from build123d import *

# Parameters (mm, degrees)
SKETCH1_R           = 3
SKETCH1_R_2         = 2.25
SKETCH1_W           = 9.525
SKETCH1_H           = 3.175
BOSS_EXTRUDE1_DEPTH = 3.175


with BuildPart() as part:
    # Sketch1 → Boss-Extrude1 (new body)
    with BuildSketch(Plane(origin=(0, 0, 0), x_dir=(1, 0, 0), z_dir=(0, 1, 0))):
        with BuildLine():
            Line((-12.7, -15.875), (101.8, -15.875))
            ThreePointArc((101.8, -15.875), (110.638834765, -12.213834765), (114.3, -3.375))
            Line((114.3, -3.375), (114.3, 3.375))
            ThreePointArc((114.3, 3.375), (110.638834765, 12.213834765), (101.8, 15.875))
            Line((101.8, 15.875), (-12.7, 15.875))
            Line((-12.7, 15.875), (-12.7, -15.875))
        make_face()
        Circle(SKETCH1_R, mode=Mode.SUBTRACT)
        with Locations((98.425, 0)):
            Circle(SKETCH1_R_2, mode=Mode.SUBTRACT)
        with Locations((50.8, 0)):
            Circle(SKETCH1_R, mode=Mode.SUBTRACT)
        with Locations((12.7, 0)):
            Rectangle(SKETCH1_W, SKETCH1_H, mode=Mode.SUBTRACT)
    extrude(amount=BOSS_EXTRUDE1_DEPTH)


solid = part.part
Verification items for the finished model (mm, model axes). A direction names the side the tool comes from. Give positions to 0.01 mm unless a question says otherwise; leave off trailing zeros. Write each loop counter-clockwise with the first axis right and the second up, starting at its lowest first coordinate (ties: lowest second). Pieces come first, ordered by that corner, then holes. Notation, with made-up numbers: M 69.5,87.5 L 76.5,87.5 A32 cw 76.5,124.5 Z; hole C 0.25,11 d5. An arc over 180 degrees is marked long. Write item = value, one per line.
(1) Sectioned sample at D-D (z = 12.5). Record the cut outline in (x, y) (3 decimals).
Found:
outline = M -12.7,0 L 110.343,0 L 110.343,3.175 L -12.7,3.175 Z
(2) Sectioned sample at B-B (z = 0). Record the cut outline in (x, y) (1 decimal).
Found:
outline = M -12.7,0 L -3,0 L -3,3.2 L -12.7,3.2 Z; M 3,0 L 7.9,0 L 7.9,3.2 L 3,3.2 Z; M 17.5,0 L 47.8,0 L 47.8,3.2 L 17.5,3.2 Z; M 53.8,0 L 96.2,0 L 96.2,3.2 L 53.8,3.2 Z; M 100.7,0 L 114.3,0 L 114.3,3.2 L 100.7,3.2 Z
(3) Access from +Z, -Z, +X, -X, +Y, -Y to the whole of each face (thin tool, end or side, straight path). Record for faces 1 (the face through (50, 3.175, -4)), 2 (the face through (7.937, 2, 0)).
Found:
face_1 = +Z, -Z, +X, -X, +Y
face_2 = +Y, -Y
(4) Draft check along X on faces 3 (the face through (45, 2, -15.875)), 4 (the face through (17.462, 2, 0)), 5 (the face through (-12.7, 2, 0)). Enter one of: released by +X, released by -X, zero draft, split by the parting line, or undercut.
Found:
face_3 = zero draft
face_4 = undercut
face_5 = released by -X
(5) Material ranges on line 1 (X direction, y = 1.5, z = 0) (1 decimal); line 2 (X direction, y = 1.15, z = -2.5); line 3 (Z direction, x = 0, y = 1.45) (3 decimals), recorded low to high.
Found:
line_1 = -12.7 to -3, 3 to 7.9, 17.5 to 47.8, 53.8 to 96.2, 100.7 to 114.3
line_2 = -12.7 to -1.66, 1.66 to 49.14, 52.46 to 114.3
line_3 = -15.875 to -3, 3 to 15.875
(6) Sectioned sample at A-A (x = 50.8). Record the cut outline in (y, z) (3 decimals).
Found:
outline = M 0,-15.875 L 3.175,-15.875 L 3.175,-3 L 0,-3 Z; M 0,3 L 3.175,3 L 3.175,15.875 L 0,15.875 Z
(7) Sectioned sample at C-C (y = 1.3). Give the number of separate pieces and of enclosed holes in the cut face, then the cut area to 3 significant figures.
Found:
separate_pieces = 1
enclosed_holes = 4
area = 3,860 mm2
(8) Go/stop test with a flat-tipped pin: pin 1 Ø5 at (x, z) = (0, 0) entering from +Y. Record where the tip stops, or that it passes through.
Found:
pin_1 = through
